from build123d import *

# Parameters (mm, degrees)
F1_DEPTH = 12.7


with BuildPart() as f1:
    # F0 (on Front) → F1 (new body)
    with BuildSketch(Plane.XZ):
        Polygon((40.453546, 15.269228), (0, 54.136354), (-40.85014, 15.269228), align=None)
        Polygon((40.453546, 15.269228), (-40.85014, 15.269228), (-40.85014, -36.685806), (0, -56.912575), (41.643355, -35.892602), align=None)
    extrude(amount=F1_DEPTH)


solid = f1.part
Can you work these out from the model? Positions are in its coordinate system, mm. Coordinates: 2 decimals unless noted, no trailing zeros. Loops run counter-clockwise (first coordinate to the right, second up) from the corner with the lowest first, then second, coordinate; pieces in that order, holes last. Notation, with made-up numbers: (-11, 20) - (18, 20) arc R27 ccw to (18, 45) - close; hole circle Ø8 at (-36.5, 17). An arc over 180 degrees is marked (long way). Put each result on its own line as item: value. Start each with the question number.
Item 1: Suppose I cut it at B-B (x = 23). Please give me the cut outline in (y, z), and give its area (3 significant figures).
Item 2: Suppose I cut it at C-C (z = 47). Please give me the cut outline in (x, y), and give its area (3 significant figures).
Item 3: For pin 1 (1.5 mm diameter, centred on x = -32, y = -7, fed in from +Z); pin 2 (1 mm diameter, centred on x = -18, y = -10, fed in from +Z), each with a flat end and sliding along its axis, tell me the tip position at first contact or that it passes through.
Item 4: Suppose I cut it at A-A (y = -10.5). Please give me the cut outline in (x, z).
Item 5: If I drill on line 1 along X through (y, z) = (-11.5, 14.5); line 2 along Z through (x, y) = (16.5, -9.5); line 3 along X through (y, z) = (-0.25, -15), over which ranges is the centre line in solid material (lowest first)?
Here are the results:
1. outline: (-12.7, -45.3) - (0, -45.3) - (0, 32.04) - (-12.7, 32.04) - close
1. area: 982 mm²
2. outline: (-7.5, -12.7) - (7.43, -12.7) - (7.43, 0) - (-7.5, 0) - close
2. area: 190 mm²
3. pin 1: z = 24.4
3. pin 2: z = 37.49
4. outline: (-40.85, -36.69) - (0, -56.91) - (41.64, -35.89) - (40.45, 15.27) - (0, 54.14) - (-40.85, 15.27) - close
5. line 1: -40.85 to 40.47
5. line 2: -48.58 to 38.28
5. line 3: -40.85 to 41.16
